Could you check a few things on this model? Use its own coordinates, in mm. A direction names the side the tool comes from. Give positions to 0.01 mm unless a question says otherwise; leave off trailing zeros. Loops run counter-clockwise (first coordinate to the right, second up) from the corner with the lowest first, then second, coordinate; pieces in that order, holes last. Notation, with made-up numbers: (-2, 16) - (38, 16) arc R20 cw to (38, 40) - close; hole circle Ø3 at (20.25, 58.25). An arc over 180 degrees is marked (long way). Write each question's results on one line, items separated by ' | '. Start each with the question number.
1) If we mould it in two halves opening along Z, with no side actions, what happens to faces 1 (the face through (-23, 30, 9)), 2 (the face through (-10, 36, 0)), 3 (the face through (-8, 39, 0)), 4 (the face through (-27.15, 30, 7))? For each: +Z half, -Z half, draft (parallel to the pull), parting line (faces both ways), or undercut.
2) I want a section at A-A, the plane x = -24.75. Write out the boundary of the cut face in (y, z), and give its area (3 significant figures).
3) I want a section at C-C, the plane y = 15. Write out the boundary of the cut face in (x, z), and give its area (3 significant figures).
4) I'm going to push flat-ended pins straight in: pin 1 (12 mm diameter, centred on y = 5.5, z = 6.5, fed in from -X); pin 2 (5.5 mm diameter, centred on x = 23, z = -3, fed in from +Y); pin 3 (8 mm diameter, centred on x = 24.75, z = 4.95, fed in from -Y). Where does each tip first touch, or does it pass through?
5) On a 3-axis mill with a long thin cutter (end or side, diameter ignored), from which of +Z, -Z, +X, -X, +Y, -Y can I reach the whole of each face in a straight line? I mean faces 5 (the face through (-23, 28.5, 0)), 6 (the face through (-23, 32.5, 0)), 7 (the face through (23, 30, -9)), 8 (the face through (0, 0, 0)), 9 (the face through (23, 32.5, 0)). Say none if no direction works.
6) I want a section at B-B, the plane y = 38.5. Write out the boundary of the cut face in (x, z), and give its area (3 significant figures).
7) If I drill on probe 1 along Z at (x, y) = (24.75, 31.7); probe 2 along X at (y, z) = (38.7, 0); probe 3 along X at (y, z) = (31, 7.25), over which ranges is the centre line in solid material (lowest first)? Write a range as [from, to].
from build123d import *

# Parameters (mm, degrees)
SKETCH1_W           = 40.2
SKETCH1_H           = 20
BOSS_EXTRUDE1_DEPTH = 40.5
SKETCH2_W           = 18
SKETCH2_H           = 2
BOSS_EXTRUDE2_DEPTH = 7.05
SKETCH5_R           = 3
CUT_EXTRUDE1_DEPTH  = 7.05
MIRROR2_START       = 28.5
MIRROR2_DEPTH       = 4
FILLET2_R           = 0.75
SKETCH6_R           = 6
BOSS_EXTRUDE3_DEPTH = 0.5
BOSS_EXTRUDE3_TAPER = 15
SKETCH7_R           = 2
CUT_EXTRUDE3_DEPTH  = 5


# Read off the part's stored shape, not the designer's step: Mirror2
with BuildPart() as part:
    # Sketch1 → Boss-Extrude1 (new body)
    with BuildSketch(Plane(origin=(0, 0, 0), x_dir=(1, 0, 0), z_dir=(0, 1, 0))):
        Rectangle(SKETCH1_W, SKETCH1_H)
    extrude(amount=BOSS_EXTRUDE1_DEPTH)

    # Sketch2 → Boss-Extrude2 (add)
    with BuildSketch(Plane(origin=(20.1, 0, 0), x_dir=(0, 0, -1), z_dir=(1, 0, 0))):
        with Locations((0, 29.5)):
            Rectangle(SKETCH2_W, SKETCH2_H)
    extrude(amount=BOSS_EXTRUDE2_DEPTH)

    # Sketch5 → Cut-Extrude1 (cut)
    with BuildSketch(Plane(origin=(0, 30.5, 0), x_dir=(1, 0, 0), z_dir=(0, 1, 0))):
        with Locations((24.75, 4.95)):
            Circle(SKETCH5_R)
        with Locations((24.75, -4.95)):
            Circle(SKETCH5_R)
    extrude(amount=-CUT_EXTRUDE1_DEPTH, mode=Mode.SUBTRACT)

    # Mirror2 outline → Mirror2 (add)
    with BuildSketch(Plane(origin=(0, 0, 0), x_dir=(1, 0, 0), z_dir=(0, 1, 0)).offset(MIRROR2_START)):
        with BuildLine():
            Line((-27.15, 3.15), (-27.15, -3.15))
            ThreePointArc((-27.15, -3.15), (-21.75, -4.95), (-27.15, -6.75))
            Line((-27.15, -6.75), (-27.15, -9))
            Line((-27.15, -9), (-20.1, -9))
            Line((-20.1, -9), (-20.1, 9))
            Line((-20.1, 9), (-27.15, 9))
            Line((-27.15, 9), (-27.15, 6.75))
            ThreePointArc((-27.15, 6.75), (-21.75, 4.95), (-27.15, 3.15))
        make_face()
        with BuildLine():
            Line((27.15, 6.75), (27.15, 9))
            Line((27.15, 9), (20.1, 9))
            Line((20.1, 9), (20.1, -9))
            Line((20.1, -9), (27.15, -9))
            Line((27.15, -9), (27.15, -6.75))
            ThreePointArc((27.15, -6.75), (21.75, -4.95), (27.15, -3.15))
            Line((27.15, -3.15), (27.15, 3.15))
            ThreePointArc((27.15, 3.15), (21.75, 4.95), (27.15, 6.75))
        make_face()
    extrude(amount=MIRROR2_DEPTH)

    # Fillet2
    fillet2_edges = [part.edges().sort_by_distance(p)[0] for p in [
        (27.15, 30.5, 9),
        (27.15, 30.5, -9),
        (-27.15, 30.5, 9),
        (-27.15, 30.5, -9),
        (20.1, 20.25, 10),
        (-20.1, 20.25, 10),
        (-20.1, 20.25, -10),
        (20.1, 20.25, -10),
    ]]
    fillet(fillet2_edges, radius=FILLET2_R)

    # Sketch6 → Boss-Extrude3 (add)
    with BuildSketch(Plane(origin=(0, 40.5, 0), x_dir=(1, 0, 0), z_dir=(0, 1, 0))):
        with Locations((-10, 0)):
            Circle(SKETCH6_R)
    extrude(amount=BOSS_EXTRUDE3_DEPTH, taper=BOSS_EXTRUDE3_TAPER)

    # Sketch7 → Cut-Extrude3 (cut)
    with BuildSketch(Plane(origin=(0, 41, 0), x_dir=(1, 0, 0), z_dir=(0, 1, 0))):
        with Locations(Location((-10, 0, 0), (0, 0, 270))):
            Circle(SKETCH7_R)
    extrude(amount=-CUT_EXTRUDE3_DEPTH, mode=Mode.SUBTRACT)


solid = part.part
Answers:
1) face 1: +Z half | face 2: undercut | face 3: undercut | face 4: draft
2) outline: (28.5, -9) - (32.5, -9) - (32.5, -7.95) - (28.5, -7.95) - close; (28.5, -1.95) - (32.5, -1.95) - (32.5, 1.95) - (28.5, 1.95) - close; (28.5, 7.95) - (32.5, 7.95) - (32.5, 9) - (28.5, 9) - close | area: 24.0 mm2
3) outline: (-20.1, -9.25) arc R0.75 ccw to (-19.35, -10) - (19.35, -10) arc R0.75 ccw to (20.1, -9.25) - (20.1, 9.25) arc R0.75 ccw to (19.35, 10) - (-19.35, 10) arc R0.75 ccw to (-20.1, 9.25) - close | area: 804 mm2
4) pin 1: stops at x = -20.1 | pin 2: stops at y = 32.5 | pin 3: stops at y = 28.5
5) face 5: +Z, -Z, -X, -Y | face 6: +Z, -Z, -X, +Y | face 7: -Z, +X, +Y, -Y | face 8: +Z, -Z, +X, -X, -Y | face 9: +Z, -Z, +X, +Y
6) outline: (-20.1, -9.25) arc R0.75 ccw to (-19.35, -10) - (19.35, -10) arc R0.75 ccw to (20.1, -9.25) - (20.1, 9.25) arc R0.75 ccw to (19.35, 10) - (-19.35, 10) arc R0.75 ccw to (-20.1, 9.25) - close; hole circle Ø4 at (-10, 0) | area: 791 mm2
7) probe 1: z = [-9, -7.95], [-1.95, 1.95], [7.95, 9] | probe 2: x = [-20.1, -12], [-8, 20.1] | probe 3: x = [-27.15, -26.68], [-22.82, 22.82], [26.68, 27.15]
